Can you work these out from the model? Positions are in its coordinate system, mm. A direction names the side the tool comes from. Give positions to 0.01 mm unless a question says otherwise; leave off trailing zeros. Loops run counter-clockwise (first coordinate to the right, second up) from the corner with the lowest first, then second, coordinate; pieces in that order, holes last. Notation, with made-up numbers: (63.25, 38.25) -> (96.25, 38.25) arc R22 cw to (96.25, 68.25) -> close; hole circle Ø10 at (32.5, -33). An arc over 180 degrees is marked (long way). Return JSON: item names as keys, results as strings. Group by question number.
Q1. Which directions (+Z, -Z, +X, -X, +Y, -Y) give clear straight access to the entire face, cutting with the end or side of a thin tool? Please do faces 1 (the cylindrical face through (67.6, 22.7, -66.7)), 2 (the cylindrical face through (-0.924, 1.711, -77.196)).
Q2. I need wall thicknesses on line 1 along X through (y, z) = (24, -70); line 2 along Z through (x, y) = (65, 30.5); line 3 along X through (y, z) = (35.5, 30.5). Which ranges of each line are inside material? Lowest first, please. Write a range as [from, to].
Q3. Suppose I cut it at A-A, the plane y = 38.5. Count the separate pieces of the cut face and the enclosed holes in it, and give its area (3 significant figures).
Q4. Will these pins go through, and if not, where does the flat tip stop? pin 1 (1.5 mm diameter, centred on x = 53, z = -32.5, fed in from +Y); pin 2 (0.6 mm diameter, centred on x = -73.5, z = 47, fed in from -Y); pin 3 (1 mm diameter, centred on x = 72.5, z = -10, fed in from -Y).
Q5. Thinking about a two-plate mould opening in X: for faces 3 (the cylindrical face through (-71.719, 26.706, 76.594)), 4 (the flat face through (72, 24.7, 1)), 5 (the cylindrical face through (71.594, 26.706, 76.719)), which applies, pulls with the +X half, pulls with the -X half, needs draft (parallel to the pull), parting line crosses it, or undercut?
Q6. Suppose I cut it at D-D, the plane x = -36. Please give me the cut outline in (y, z), and give its area (3 significant figures).
Q7. Suppose I cut it at C-C, the plane z = 19.5. Please give me the cut outline in (x, y), and give its area (3 significant figures).
```python
from build123d import *

# Parameters (mm, degrees)
BOSS_EXTRUDE1_DEPTH = 2
BOSS_EXTRUDE2_DEPTH = 46
SKETCH5_R           = 4.2
SKETCH5_R_2         = 1.25
BOSS_EXTRUDE3_DEPTH = 42
FILLET1_R           = 6
SKETCH7_W           = 18
SKETCH7_H           = 12
SKETCH7_W_2         = 26
SKETCH7_H_2         = 18
CUT_EXTRUDE5_DEPTH  = 2
SKETCH9_W           = 6
SKETCH9_H           = 3
CUT_EXTRUDE7_DEPTH  = 2
SKETCH10_W          = 64
SKETCH10_H          = 28
CUT_EXTRUDE8_DEPTH  = 2
SKETCH11_W          = 3
SKETCH11_H          = 34
CUT_EXTRUDE9_DEPTH  = 2


with BuildPart() as part:
    # Sketch3 → Boss-Extrude1 (new body)
    with BuildSketch(Plane(origin=(0, 0, 0), x_dir=(1, 0, 0), z_dir=(0, 1, 0))):
        with BuildLine():
            Line((-66, -79), (66, -79))
            ThreePointArc((66, -79), (71.656854249, -76.656854249), (74, -71))
            Line((74, -71), (74, 71))
            ThreePointArc((74, 71), (71.656854249, 76.656854249), (66, 79))
            Line((66, 79), (-66, 79))
            ThreePointArc((-66, 79), (-71.656854249, 76.656854249), (-74, 71))
            Line((-74, 71), (-74, -71))
            ThreePointArc((-74, -71), (-71.656854249, -76.656854249), (-66, -79))
        make_face()
    extrude(amount=BOSS_EXTRUDE1_DEPTH)

    # Sketch4 → Boss-Extrude2 (add)
    with BuildSketch(Plane(origin=(0, 2, 0), x_dir=(1, 0, 0), z_dir=(0, 1, 0))):
        with BuildLine():
            Line((-66, -79), (66, -79))
            ThreePointArc((66, -79), (71.656854249, -76.656854249), (74, -71))
            Line((74, -71), (74, 71))
            ThreePointArc((74, 71), (71.656854249, 76.656854249), (66, 79))
            Line((66, 79), (-66, 79))
            ThreePointArc((-66, 79), (-71.656854249, 76.656854249), (-74, 71))
            Line((-74, 71), (-74, -71))
            ThreePointArc((-74, -71), (-71.656854249, -76.656854249), (-66, -79))
        make_face()
        with BuildLine():
            Line((-66, -77), (66, -77))
            ThreePointArc((66, -77), (70.242640687, -75.242640687), (72, -71))
            Line((72, -71), (72, 71))
            ThreePointArc((72, 71), (70.242640687, 75.242640687), (66, 77))
            Line((66, 77), (-66, 77))
            ThreePointArc((-66, 77), (-70.242640687, 75.242640687), (-72, 71))
            Line((-72, 71), (-72, -71))
            ThreePointArc((-72, -71), (-70.242640687, -75.242640687), (-66, -77))
        make_face(mode=Mode.SUBTRACT)
    extrude(amount=BOSS_EXTRUDE2_DEPTH)

    # Sketch5 → Boss-Extrude3 (add)
    # profile 1 of 4: a face of its own
    with BuildSketch(Plane(origin=(0, 2, 0), x_dir=(1, 0, 0), z_dir=(0, 1, 0))):
        with Locations(Location((-65, 70, 0), (0, 0, 90))):
            Circle(SKETCH5_R)
        with Locations(Location((-65, 70, 0), (0, 0, 90))):
            Circle(SKETCH5_R_2, mode=Mode.SUBTRACT)
    # profile 2 of 4: a face of its own
    with BuildSketch(Plane(origin=(0, 2, 0), x_dir=(1, 0, 0), z_dir=(0, 1, 0))):
        with Locations(Location((65, 70, 0), (0, 0, 90))):
            Circle(SKETCH5_R)
        with Locations(Location((65, 70, 0), (0, 0, 90))):
            Circle(SKETCH5_R_2, mode=Mode.SUBTRACT)
    # profile 3 of 4: a face of its own
    with BuildSketch(Plane(origin=(0, 2, 0), x_dir=(1, 0, 0), z_dir=(0, 1, 0))):
        with Locations(Location((65, -70, 0), (0, 0, 90))):
            Circle(SKETCH5_R)
        with Locations(Location((65, -70, 0), (0, 0, 90))):
            Circle(SKETCH5_R_2, mode=Mode.SUBTRACT)
    # profile 4 of 4: a face of its own
    with BuildSketch(Plane(origin=(0, 2, 0), x_dir=(1, 0, 0), z_dir=(0, 1, 0))):
        with Locations(Location((-65, -70, 0), (0, 0, 90))):
            Circle(SKETCH5_R)
        with Locations(Location((-65, -70, 0), (0, 0, 90))):
            Circle(SKETCH5_R_2, mode=Mode.SUBTRACT)
    extrude(amount=BOSS_EXTRUDE3_DEPTH)

    # Fillet1
    fillet1_edges = [part.edges().sort_by_distance(p)[0] for p in [
        (0, 0, -79),
        (71.656854249, 0, -76.656854249),
        (74, 0, 0),
        (71.656854249, 0, 76.656854249),
        (0, 0, 79),
        (-71.656854249, 0, 76.656854249),
        (-74, 0, 0),
        (-71.656854249, 0, -76.656854249),
    ]]
    fillet(fillet1_edges, radius=FILLET1_R)

    # Sketch7 → Cut-Extrude5 (cut)
    with BuildSketch(Plane.ZY.offset(74)):
        with Locations((50, 26)):
            Rectangle(SKETCH7_W, SKETCH7_H)
        with Locations((-45, 24)):
            Rectangle(SKETCH7_W_2, SKETCH7_H_2)
    extrude(amount=-CUT_EXTRUDE5_DEPTH, mode=Mode.SUBTRACT)

    # Sketch9 → Cut-Extrude7 (cut)
    with BuildSketch(Plane(origin=(74, 0, 0), x_dir=(0, 0, -1), z_dir=(1, 0, 0))):
        with Locations((0, 33.5)):
            Rectangle(SKETCH9_W, SKETCH9_H)
        with Locations((0, 26.5)):
            Rectangle(SKETCH9_W, SKETCH9_H)
        with Locations((-10, 33.5)):
            Rectangle(SKETCH9_W, SKETCH9_H)
        with Locations((-10, 26.5)):
            Rectangle(SKETCH9_W, SKETCH9_H)
        with Locations((-20, 26.5)):
            Rectangle(SKETCH9_W, SKETCH9_H)
        with Locations((-20, 33.5)):
            Rectangle(SKETCH9_W, SKETCH9_H)
        with Locations((20, 33.5)):
            Rectangle(SKETCH9_W, SKETCH9_H)
        with Locations((20, 26.5)):
            Rectangle(SKETCH9_W, SKETCH9_H)
        with Locations((10, 26.5)):
            Rectangle(SKETCH9_W, SKETCH9_H)
        with Locations((10, 33.5)):
            Rectangle(SKETCH9_W, SKETCH9_H)
    extrude(amount=-CUT_EXTRUDE7_DEPTH, mode=Mode.SUBTRACT)

    # Sketch10 → Cut-Extrude8 (cut)
    with BuildSketch(Plane.XY.offset(79)):
        with Locations((0, 34)):
            Rectangle(SKETCH10_W, SKETCH10_H)
    extrude(amount=-CUT_EXTRUDE8_DEPTH, mode=Mode.SUBTRACT)

    # Sketch11 → Cut-Extrude9 (cut)
    with BuildSketch(Plane.XZ):
        with Locations((58, 0)):
            Rectangle(SKETCH11_W, SKETCH11_H)
        with Locations((46, 0)):
            Rectangle(SKETCH11_W, SKETCH11_H)
        with Locations((52, 0)):
            Rectangle(SKETCH11_W, SKETCH11_H)
        with Locations((40, 0)):
            Rectangle(SKETCH11_W, SKETCH11_H)
        with Locations((34, 0)):
            Rectangle(SKETCH11_W, SKETCH11_H)
        with Locations((28, 0)):
            Rectangle(SKETCH11_W, SKETCH11_H)
    extrude(amount=-CUT_EXTRUDE9_DEPTH, mode=Mode.SUBTRACT)


solid = part.part
```
Ans:
{
 "1": {"face 1": "+Y", "face 2": "-Z, +X, -X, -Y"},
 "2": {"line 1": "x = [-74, -72], [-69.2, -66.25], [-63.75, -60.8], [60.8, 63.75], [66.25, 69.2], [72, 74]", "line 2": "z = [-79, -77], [-74.2, -71.25], [-68.75, -65.8], [65.8, 68.75], [71.25, 74.2], [77, 79]", "line 3": "x = [-74, -72], [72, 74]"},
 "3": {"separate pieces": "5", "enclosed holes": "4", "area": "1,260 mm^2"},
 "4": {"pin 1": "stops at y = 2", "pin 2": "stops at y = 3.01", "pin 3": "stops at y = 1.53"},
 "5": {"face 3": "pulls with the -X half", "face 4": "undercut", "face 5": "pulls with the +X half"},
 "6": {"outline": "(0, -73) arc R6 ccw to (6, -79) -> (48, -79) -> (48, -77) -> (2, -77) -> (2, 77) -> (48, 77) -> (48, 79) -> (6, 79) arc R6 ccw to (0, 73) -> close", "area": "485 mm^2"},
 "7": {"outline": "(-74, 6) arc R6 ccw to (-68, 0) -> (68, 0) arc R6 ccw to (74, 6) -> (74, 25) -> (72, 25) -> (72, 2) -> (-72, 2) -> (-72, 48) -> (-74, 48) -> close; (72, 28) -> (74, 28) -> (74, 32) -> (72, 32) -> close; (72, 35) -> (74, 35) -> (74, 48) -> (72, 48) -> close", "area": "453 mm^2"}
}
